Geometry check sheet. Reference: the model listing, model coordinates, mm. Face numbers are marked on the shaded views. Round coordinates to 2 decimals unless told otherwise and drop trailing zeros. Loops run counter-clockwise (first coordinate to the right, second up) from the corner with the lowest first, then second, coordinate; pieces in that order, holes last. Notation, with made-up numbers: (29.25, 71.25) - (65.25, 71.25) arc R26 ccw to (65.25, 99.25) - close; hole circle Ø4 at (-27, -16.5). An arc over 180 degrees is marked (long way). Answer as CSV lines item,"result". Start each with the question number.
1) Cross-section at A-A on z = 14.5. Record the boundary of the cut face in (x, y).
2) Depth check by flat-ended pin: P1, Ø2, axis at y = 5.5, z = 58, coming from the -X side; P2, Ø2, axis at y = 7, z = 52, coming from the +X side; P3, Ø1, axis at x = -134, y = 4, coming from the -Z side. Enter the tip coordinate at first touch or a pass-through.
3) Thickness scan on line 1 along X through (y, z) = (4.5, 62.5); line 2 along X through (y, z) = (3.75, 9); line 3 along Y through (x, z) = (-102, 18.5). Record the ranges inside material, lowest first.
4) Cross-section at D-D on z = 66.5. Record the boundary of the cut face in (x, y), and give its area (3 significant figures).
5) Cross-section at C-C on x = -53. Record the boundary of the cut face in (y, z), and give its area (3 significant figures).
6) Draft check along X on the marked faces 1 and 2. Enter one of: released by +X, released by -X, zero draft, split by the parting line, or undercut.
from build123d import *

# Parameters (mm, degrees)
F1_DEPTH = 5
F5_DEPTH = 7.5
F6_DEPTH = 2.5
F7_DEPTH = 5
F3_R     = 1.25
F4_R     = 1.25
F8_DEPTH = 1.5
F9_DEPTH = 1.5
F10_R    = 1


with BuildPart() as f1:
    # F0 (on Front) → F1 (new body)
    with BuildSketch(Plane.XZ):
        Polygon((-135.5, 0), (0, 0), (135.5, 0), (135.5, 18), (132, 18), (132, 160), (-132, 160), (-132, 18), (-135.5, 18), align=None)
    extrude(amount=-F1_DEPTH)

    # F2 (on face) → F5 (join)
    with BuildSketch(Plane.XZ):
        Polygon((-138.55, 0), (-135.55, 0), (-135.55, 18.05), (-132.05, 18.05), (-132.05, 94.05), (132.05, 94.05), (132.05, 18.05), (135.55, 18.05), (135.55, 0), (138.55, 0), (138.55, 21.05), (135, 21.05), (135, 97.05), (-135, 97.05), (-135, 21.05), (-138.55, 21.05), align=None)
    extrude(amount=-F5_DEPTH)

    # F6 (add): a face of the model
    f6_faces = [f1.faces().sort_by_distance(p)[0] for p in [
        (0, 5, 46.8330099538),
    ]]
    extrude(f6_faces, amount=F6_DEPTH)

    # F0 (on Front) → F7 (cut)
    with BuildSketch(Plane.XZ):
        Polygon((-135.5, 0), (0, 0), (135.5, 0), (135.5, 18), (132, 18), (132, 160), (-132, 160), (-132, 18), (-135.5, 18), align=None)
    extrude(amount=-F7_DEPTH, mode=Mode.SUBTRACT)

    # F3 (on face) + F4 (on face) → F8 (join)
    with BuildSketch(Plane.YZ.offset(132)):
        with Locations((2.5, 89)):
            Circle(F3_R)
    with BuildSketch(Plane(origin=(-132, 0, 0), x_dir=(0, -1, 0), z_dir=(-1, 0, 0))):
        with Locations((-2.5, 89)):
            Circle(F4_R)
    extrude(amount=F8_DEPTH, dir=(1, 0, 0))

    # F3 (on face) + F4 (on face) → F9 (join)
    with BuildSketch(Plane.YZ.offset(132)):
        with Locations((2.5, 89)):
            Circle(F3_R)
    with BuildSketch(Plane(origin=(-132, 0, 0), x_dir=(0, -1, 0), z_dir=(-1, 0, 0))):
        with Locations((-2.5, 89)):
            Circle(F4_R)
    extrude(amount=-F9_DEPTH, dir=(1, 0, 0))

    # F10
    f10_edges = [f1.edges().sort_by_distance(p)[0] for p in [
        (-135, 0, 59.05),
        (-135, 7.5, 59.05),
        (135, 7.5, 59.05),
        (135, 0, 59.05),
        (135, 3.75, 97.05),
        (0, 7.5, 97.05),
        (-135, 3.75, 97.05),
        (-136.775, 0, 21.05),
        (-136.775, 7.5, 21.05),
        (-138.55, 3.75, 21.05),
        (-138.55, 0, 10.525),
        (-138.55, 7.5, 10.525),
        (-138.55, 3.75, 0),
        (0, 7.5, 0),
        (-137.05, 7.5, 0),
        (137.05, 7.5, 0),
        (138.55, 7.5, 10.525),
        (138.55, 3.75, 0),
        (138.55, 0, 10.525),
        (138.55, 3.75, 21.05),
        (136.775, 0, 21.05),
        (136.775, 7.5, 21.05),
        (133.5, 0, 97.05),
        (-133.5, 0, 97.05),
    ]]
    fillet(f10_edges, radius=F10_R)


solid = f1.part
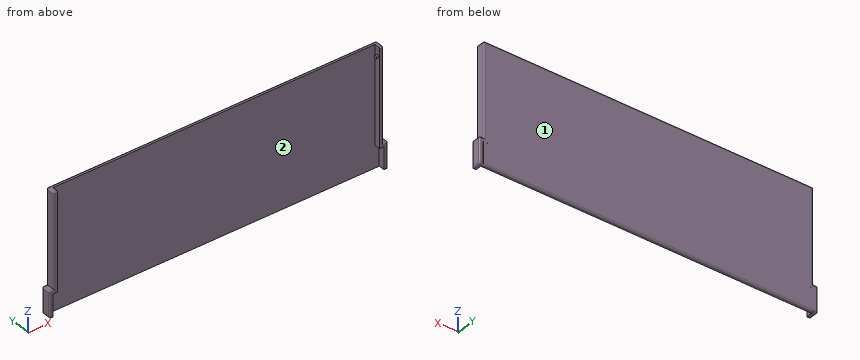
Answer block:
1,outline,"(-138.55, 1) arc R1 ccw to (-137.55, 0) - (-135.55, 0) - (-135.55, 7.5) - (-137.55, 7.5) arc R1 ccw to (-138.55, 6.5) - close; (-135.5, 5) - (135.5, 5) - (135.5, 7.5) - (-135.5, 7.5) - close; (135.55, 0) - (137.55, 0) arc R1 ccw to (138.55, 1) - (138.55, 6.5) arc R1 ccw to (137.55, 7.5) - (135.55, 7.5) - close"
2,P1,"stops at x = -135"
2,P2,"stops at x = 135"
2,P3,"stops at z = 18.05"
3,line 1,"x = -135 to -132.05, 132.05 to 135"
3,line 2,"x = -138.55 to -135.55, 135.55 to 138.55"
3,line 3,"y = 5 to 7.5"
4,outline,"(-135, 1) arc R1 ccw to (-134, 0) - (-132.05, 0) - (-132.05, 7.5) - (-134, 7.5) arc R1 ccw to (-135, 6.5) - close; (-132, 5) - (132, 5) - (132, 7.5) - (-132, 7.5) - close; (132.05, 0) - (134, 0) arc R1 ccw to (135, 1) - (135, 6.5) arc R1 ccw to (134, 7.5) - (132.05, 7.5) - close"
4,area,"703 mm^2"
5,outline,"(5, 0) - (6.5, 0) arc R1 ccw to (7.5, 1) - (7.5, 96.05) arc R1 ccw to (6.5, 97.05) - (5, 97.05) - close"
5,area,"242 mm^2"
6,face 1,"zero draft"
6,face 2,"undercut"
